For this review, use the dimensioned drawing (mm, ordinates from the lowest corner) and the shaded views. A direction names the side the tool comes from. Coordinates: 2 decimals unless noted, no trailing zeros. Write each loop counter-clockwise with the first axis right and the second up, starting at its lowest first coordinate (ties: lowest second). Pieces come first, ordered by that corner, then holes. Notation, with made-up numbers: M -32,40.5 L 7,40.5 A24 ccw 7,68.5 Z; hole C -34.5,43.5 d11. An arc over 180 degrees is marked long. Return JSON: item names as keys, results as strings. Group by question number.
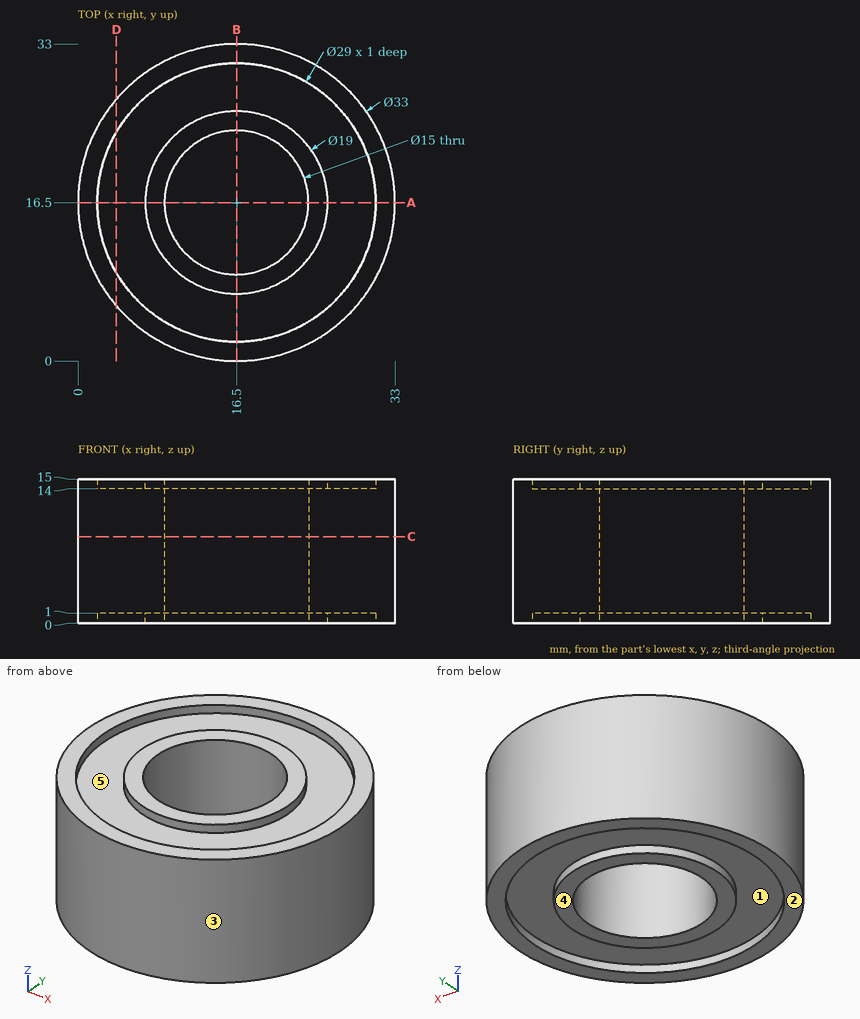
Item 1: The part is to be moulded in two halves that separate along X. For the marked faces 1, 2 and 3, say which applies: pulls with the +X half, pulls with the -X half, needs draft (parallel to the pull), parting line crosses it, or undercut.
Item 2: Machinability: for the marked faces 4 and 5, which of the approach directions +Z, -Z, +X, -X, +Y, -Y give a long, thin tool a straight path to every point of the face, cutting with its end or side? Answer none if there is none.
Item 3: Add section C-C (z = 9). Write out the cut boundary in (x, y), plus the area to 3 significant figures.
Item 4: Add section A-A (y = 16.5). Write out the cut boundary in (x, z).
Item 5: Add section D-D (x = 4). Write out the cut boundary in (y, z).
Item 6: For line 1 (Y direction, x = 16.5, z = 0.5); line 2 (Y direction, x = 16.5, z = 7.5); line 3 (X direction, y = 11.5, z = 4.5), list the stretches that pass through material, from the lowest coordinate up.
Item 7: For pin 1 (1.5 mm diameter, centred on x = 8, z = 10.5, fed in from -Y); pin 2 (3 mm diameter, centred on y = 12.5, z = 12, fed in from -X); pin 3 (4 mm diameter, centred on x = 4.5, z = 8.5, fed in from +Y), all flat-tipped, find the tip position at first contact; note any pin that passes through.
Geometry check:
{
 "1": {"face 1": "undercut", "face 2": "needs draft", "face 3": "parting line crosses it"},
 "2": {"face 4": "-Z, +X, -X, +Y, -Y", "face 5": "+Z"},
 "3": {"outline": "C 16.5,16.5 d33; hole C 16.5,16.5 d15", "area": "679 mm^2"},
 "4": {"outline": "M 0,0 L 2,0 L 2,1 L 7,1 L 7,0 L 9,0 L 9,15 L 7,15 L 7,14 L 2,14 L 2,15 L 0,15 Z; M 24,0 L 26,0 L 26,1 L 31,1 L 31,0 L 33,0 L 33,15 L 31,15 L 31,14 L 26,14 L 26,15 L 24,15 Z"},
 "5": {"outline": "M 5.73,0 L 9.15,0 L 9.15,1 L 23.85,1 L 23.85,0 L 27.27,0 L 27.27,15 L 23.85,15 L 23.85,14 L 9.15,14 L 9.15,15 L 5.73,15 Z"},
 "6": {"line 1": "0 to 2, 7 to 9, 24 to 26, 31 to 33", "line 2": "0 to 9, 24 to 33", "line 3": "0.78 to 10.91, 22.09 to 32.22"},
 "7": {"pin 1": "y = 1.93", "pin 2": "x = 0.19", "pin 3": "y = 29.62"}
}
